Read the model definition and answer for the solid it produces. Units are mm, in the model's axes. A direction names the side the tool comes from. Coordinates: 2 decimals unless noted, no trailing zeros. Write each loop counter-clockwise with the first axis right and the second up, starting at its lowest first coordinate (ties: lowest second). Pieces come first, ordered by that corner, then holes. Notation, with made-up numbers: (-30.75, 19.5) -> (19.25, 19.5) arc R26 ccw to (19.25, 38.5) -> close; hole circle Ø8 at (-16.5, 73.5). An arc over 180 degrees is marked (long way). Answer in a Markdown table with one row per item. Add a question column.
Item 1: Section B-B on x = 15 is taken. Write down the section's boundary in (y, z).
Item 2: Which of the six approach directions +Z, -Z, +X, -X, +Y, -Y give full straight-line access (tool end or side, diameter ignored) to faces 1 (the face through (6.89, 57.88, -16.01)), 2 (the face through (15, 29, -29.569)), 3 (the face through (26.01, -0.74, -26.11))?
Item 3: For a pull along Z with two mould halves and no side action, classify faces 4 (the face through (15, 58, 0)), 5 (the face through (20.5, 57.88, -15.07)), 6 (the face through (15, 58.638, -15)), 7 (the face through (5.07, -0.74, -6.5)) as +Z half, -Z half, draft (parallel to the pull), parting line (faces both ways), or undercut.
Item 4: Straight lines are drawn through the part: line 1 (Y direction, x = 4.5, z = -21); line 2 (X direction, y = -1.05, z = -25); line 3 (Z direction, x = 17.25, y = 49). For each, find the intervals that lie inside material, in ascending order. Write a range as from..to.
Item 5: Section C-C on z = -25 is taken. Write down the section's boundary in (x, y), then the cut area to 3 significant figures.
Item 6: Section A-A on z = -15 is taken. Write down the section's boundary in (x, y), then the cut area to 3 significant figures.
Item 7: Given pin 1 Ø15 at (x, y) = (14, 27.5) entering from +Z; pin 2 Ø2.5 at (x, z) = (5, -5) entering from -Y, each flat-ended and moving along its own axis, determine where each tip first touches the part or whether it passes through.
Item 8: Section D-D on z = -2 is taken. Write down the section's boundary in (x, y), then the cut area to 3 significant figures.
```python
from build123d import *

# Parameters (mm, degrees)
SKETCH1_W                       = 30
SKETCH1_H                       = 118
SKETCH1_R                       = 1.5
BASE_FLANGE1_DEPTH              = 1.5
SKETCHED_BEND1_DEPTH            = 30
SKETCHED_START                  = 9.5000001
SKETCHED_BEND1_2_DEPTH          = 10.9999998
SKETCHED_BEND1_3_DEPTH          = 6.4999999
SKETCHED_START_2                = 23.5000001
SKETCHED_BEND1_4_DEPTH          = 6.4999999
SKETCHED_START_3                = 6.4999999
SKETCHED_BEND1_5_DEPTH          = 17.0000002
SKETCHED_START_4                = 57.138054181
SKETCHED_BEND1_6_OUTLINE_R      = 1.5
SKETCHED_BEND1_6_DEPTH          = 1.5
F_3_0MM_PRESS_DOWEL_HOLE1_D     = 3
F_3_0MM_PRESS_DOWEL_HOLE1_DEPTH = 6
F_3_0MM_PRESS_DOWEL_HOLE1_TIP   = 0.901290929
F_3_0MM_PRESS_DOWEL_HOLE2_D     = 3


with BuildPart() as part:
    # Base-Flange1: sheet metal written as solids
    # Sketch1 → Base-Flange1 (new body)
    with BuildSketch(Plane(origin=(0, 0, 0), x_dir=(1, 0, 0), z_dir=(0, 1, 0))):
        with Locations((15, 59)):
            Rectangle(SKETCH1_W, SKETCH1_H)
        with Locations(Location((8, 103, 0), (0, 0, 270))):
            Circle(SKETCH1_R, mode=Mode.SUBTRACT)
        with Locations(Location((22, 103, 0), (0, 0, 270))):
            Circle(SKETCH1_R, mode=Mode.SUBTRACT)
        with Locations(Location((25, 25, 0), (0, 0, 270))):
            Circle(SKETCH1_R, mode=Mode.SUBTRACT)
        with Locations(Location((5, 5, 0), (0, 0, 270))):
            Circle(SKETCH1_R, mode=Mode.SUBTRACT)
    extrude(amount=-BASE_FLANGE1_DEPTH)

    # Sketched Bend1: read off the stored shape, not the designer's step
    # Sketched Bend1 outline → Sketched Bend1 (cut)
    with BuildSketch(Plane.YZ):
        with BuildLine():
            Line((0, -118), (0, -30.944250946))
            ThreePointArc((0, -30.944250946), (-1.086838938, -30.127591172), (-1.5, -28.83242709))
            Line((-1.5, -28.83242709), (-1.5, -118))
            Line((-1.5, -118), (0, -118))
        make_face()
    extrude(amount=SKETCHED_BEND1_DEPTH, mode=Mode.SUBTRACT)

    # Sketched Bend1 2 outline → Sketched Bend1 2 (add)
    with BuildSketch(Plane.YZ.offset(SKETCHED_START)):
        with BuildLine():
            Line((56.401454181, -29.56902709), (0.7366, -29.56902709))
            ThreePointArc((0.7366, -29.56902709), (0.215745145, -29.353281945), (0, -28.83242709))
            Line((0, -28.83242709), (0, -30.944250946))
            ThreePointArc((0, -30.944250946), (0.363053267, -31.037612433), (0.7366, -31.06902709))
            Line((0.7366, -31.06902709), (56.401454181, -31.06902709))
            ThreePointArc((56.401454181, -31.06902709), (57.982969207, -30.413942116), (58.638054181, -28.83242709))
            Line((58.638054181, -28.83242709), (58.638054181, 0))
            Line((58.638054181, 0), (57.138054181, 0))
            Line((57.138054181, 0), (57.138054181, -28.83242709))
            ThreePointArc((57.138054181, -28.83242709), (56.922309036, -29.353281945), (56.401454181, -29.56902709))
        make_face()
    extrude(amount=SKETCHED_BEND1_2_DEPTH)

    # Sketched Bend1 3 outline → Sketched Bend1 3 (add)
    with BuildSketch(Plane.YZ):
        with BuildLine():
            Line((56.401454181, -29.56902709), (0.7366, -29.56902709))
            ThreePointArc((0.7366, -29.56902709), (0.215745145, -29.353281945), (0, -28.83242709))
            Line((0, -28.83242709), (0, -30.944250946))
            ThreePointArc((0, -30.944250946), (0.363053267, -31.037612433), (0.7366, -31.06902709))
            Line((0.7366, -31.06902709), (56.401454181, -31.06902709))
            ThreePointArc((56.401454181, -31.06902709), (57.982969207, -30.413942116), (58.638054181, -28.83242709))
            Line((58.638054181, -28.83242709), (58.638054181, 0))
            Line((58.638054181, 0), (57.138054181, 0))
            Line((57.138054181, 0), (57.138054181, -28.83242709))
            ThreePointArc((57.138054181, -28.83242709), (56.922309036, -29.353281945), (56.401454181, -29.56902709))
        make_face()
    extrude(amount=SKETCHED_BEND1_3_DEPTH)

    # Sketched Bend1 4 outline → Sketched Bend1 4 (add)
    with BuildSketch(Plane.YZ.offset(SKETCHED_START_2)):
        with BuildLine():
            Line((56.401454181, -29.56902709), (0.7366, -29.56902709))
            ThreePointArc((0.7366, -29.56902709), (0.215745145, -29.353281945), (0, -28.83242709))
            Line((0, -28.83242709), (0, -30.944250946))
            ThreePointArc((0, -30.944250946), (0.363053267, -31.037612433), (0.7366, -31.06902709))
            Line((0.7366, -31.06902709), (56.401454181, -31.06902709))
            ThreePointArc((56.401454181, -31.06902709), (57.982969207, -30.413942116), (58.638054181, -28.83242709))
            Line((58.638054181, -28.83242709), (58.638054181, 0))
            Line((58.638054181, 0), (57.138054181, 0))
            Line((57.138054181, 0), (57.138054181, -28.83242709))
            ThreePointArc((57.138054181, -28.83242709), (56.922309036, -29.353281945), (56.401454181, -29.56902709))
        make_face()
    extrude(amount=SKETCHED_BEND1_4_DEPTH)

    # Sketched Bend1 5 outline → Sketched Bend1 5 (add)
    with BuildSketch(Plane.YZ.offset(SKETCHED_START_3)):
        with BuildLine():
            Line((56.401454181, -29.56902709), (0.7366, -29.56902709))
            ThreePointArc((0.7366, -29.56902709), (0.215745145, -29.353281945), (0, -28.83242709))
            Line((0, -28.83242709), (0, -30.944250946))
            ThreePointArc((0, -30.944250946), (0.363053267, -31.037612433), (0.7366, -31.06902709))
            Line((0.7366, -31.06902709), (56.401454181, -31.06902709))
            ThreePointArc((56.401454181, -31.06902709), (57.982969207, -30.413942116), (58.638054181, -28.83242709))
            Line((58.638054181, -28.83242709), (58.638054181, 0))
            Line((58.638054181, 0), (57.138054181, 0))
            Line((57.138054181, 0), (57.138054181, -28.83242709))
            ThreePointArc((57.138054181, -28.83242709), (56.922309036, -29.353281945), (56.401454181, -29.56902709))
        make_face()
    extrude(amount=SKETCHED_BEND1_5_DEPTH)

    # Sketched Bend1 6 outline → Sketched Bend1 6 (cut)
    with BuildSketch(Plane(origin=(0, 0, 0), x_dir=(1, 0, 0), z_dir=(0, 1, 0)).offset(SKETCHED_START_4)):
        with Locations((8, 15)):
            Circle(SKETCHED_BEND1_6_OUTLINE_R)
        with Locations((22, 15)):
            Circle(SKETCHED_BEND1_6_OUTLINE_R)
    extrude(amount=SKETCHED_BEND1_6_DEPTH, mode=Mode.SUBTRACT)

    # Ø3.0mm Press Dowel Hole1
    with Locations(Plane(origin=(-227.525513363, -7.5, -157.600386311), x_dir=(1, 0, 0), z_dir=(0, -1, 0))):
        with Locations((220.525513363, 156.531359221), (102.525513363, 181.531359221), (102.525513363, 271.531359221), (89.19270005, 226.531359221), (210.525513363, 317.793651488), (230.525513363, 317.793651488), (252.525513363, 320.462332131), (232.525513363, 300.462332131), (252.525513363, 132.600386311), (232.525513363, 152.600386311), (111.286271896, 136.531359221), (91.286271896, 136.531359221), (41.525513363, 196.432813402), (13.525513363, 196.432813402), (41.525513363, 138.767959221), (13.525513363, 138.767959221), (41.525513363, 256.62990504), (13.525513363, 256.62990504), (41.525513363, 314.294759221), (13.525513363, 314.294759221)):
            Hole(F_3_0MM_PRESS_DOWEL_HOLE1_D / 2, depth=F_3_0MM_PRESS_DOWEL_HOLE1_DEPTH)
            with Locations((0, 0, -(F_3_0MM_PRESS_DOWEL_HOLE1_DEPTH + F_3_0MM_PRESS_DOWEL_HOLE1_TIP / 2))):  # 118° drill point
                Cone(0, F_3_0MM_PRESS_DOWEL_HOLE1_D / 2, F_3_0MM_PRESS_DOWEL_HOLE1_TIP, mode=Mode.SUBTRACT)

    # Ø3.0mm Press Dowel Hole2 (through all)
    with Locations(Plane(origin=(0, 0, -31.06902709), x_dir=(-1, 0, 0), z_dir=(0, 0, -1))):
        with Locations((-15, 38.638054181), (-15, 18.638054181)):
            Hole(F_3_0MM_PRESS_DOWEL_HOLE2_D / 2)


solid = part.part
```
Results below:
| question | item | result |
|---|---|---|
| 1 | outline | (-1.5, -28.83) arc R2.24 ccw to (0.74, -31.07) -> (17.14, -31.07) -> (17.14, -29.57) -> (0.74, -29.57) arc R0.74 cw to (0, -28.83) -> (0, 0) -> (-1.5, 0) -> close; (20.14, -31.07) -> (37.14, -31.07) -> (37.14, -29.57) -> (20.14, -29.57) -> close; (40.14, -31.07) -> (56.4, -31.07) arc R2.24 ccw to (58.64, -28.83) -> (58.64, 0) -> (57.14, 0) -> (57.14, -28.83) arc R0.74 cw to (56.4, -29.57) -> (40.14, -29.57) -> close |
| 2 | face 1 | +Y |
| 2 | face 2 | +Z, +X, -X |
| 2 | face 3 | -Y |
| 3 | face 4 | +Z half |
| 3 | face 5 | undercut |
| 3 | face 6 | draft |
| 3 | face 7 | undercut |
| 4 | line 1 | y = -1.5..0, 57.14..58.64 |
| 4 | line 2 | x = 0..23.5, 26.5..30 |
| 4 | line 3 | z = -31.07..-29.57 |
| 5 | outline | (0, -1.5) -> (23.5, -1.5) -> (23.5, 0) -> (0, 0) -> close; (0, 57.14) -> (30, 57.14) -> (30, 58.64) -> (0, 58.64) -> close; (26.5, -1.5) -> (30, -1.5) -> (30, 0) -> (26.5, 0) -> close |
| 5 | area | 85.5 mm2 |
| 6 | outline | (0, -1.5) -> (30, -1.5) -> (30, 0) -> (0, 0) -> close; (0, 57.14) -> (6.5, 57.14) -> (6.5, 58.64) -> (0, 58.64) -> close; (9.5, 57.14) -> (20.5, 57.14) -> (20.5, 58.64) -> (9.5, 58.64) -> close; (23.5, 57.14) -> (30, 57.14) -> (30, 58.64) -> (23.5, 58.64) -> close |
| 6 | area | 81.0 mm2 |
| 7 | pin 1 | stops at z = -29.57 |
| 7 | pin 2 | stops at y = 57.14 |
| 8 | outline | (0, -1.5) -> (30, -1.5) -> (30, 0) -> (0, 0) -> close; (0, 57.14) -> (30, 57.14) -> (30, 58.64) -> (0, 58.64) -> close |
| 8 | area | 90.0 mm2 |
